Job drawing, mm, ordinate dimensions from the low corner. One solid piece. A direction names the side the tool comes from. Round coordinates to 2 decimals unless told otherwise and drop trailing zeros. Write each loop counter-clockwise with the first axis right and the second up, starting at its lowest first coordinate (ties: lowest second). Pieces come first, ordered by that corner, then holes.
1) Saw through at A-A (x = 15). Write the cut outline in (y, z).
2) Wall check: probe 1 along Z at (x, y) = (15, 26.5); probe 2 along X at (y, z) = (7, 7); probe 3 along Y at (x, z) = (1.5, 4.5). Give the ranges that are in metal, low to high.
3) Which spindle directions (+Z, -Z, +X, -X, +Y, -Y) get a long thin tool onto all of the face, cutting with end or side? Do the marked faces 1 and 2. Say none if no direction does.
4) Saw through at B-B (z = 34.5). Write the cut outline in (x, y), plus the area to 3 significant figures.
5) Saw through at C-C (y = 29). Write the cut outline in (x, z).
6) Flat gauge pins, fed straight in: pin 1 (5.5 mm diameter, centred on x = 11, z = 18, fed in from -Y); pin 2 (12 mm diameter, centred on y = 14.5, z = 12.5, fed in from -X). Where does each tip first touch, or does it go through?
7) Saw through at D-D (z = 29). Write the cut outline in (x, y).
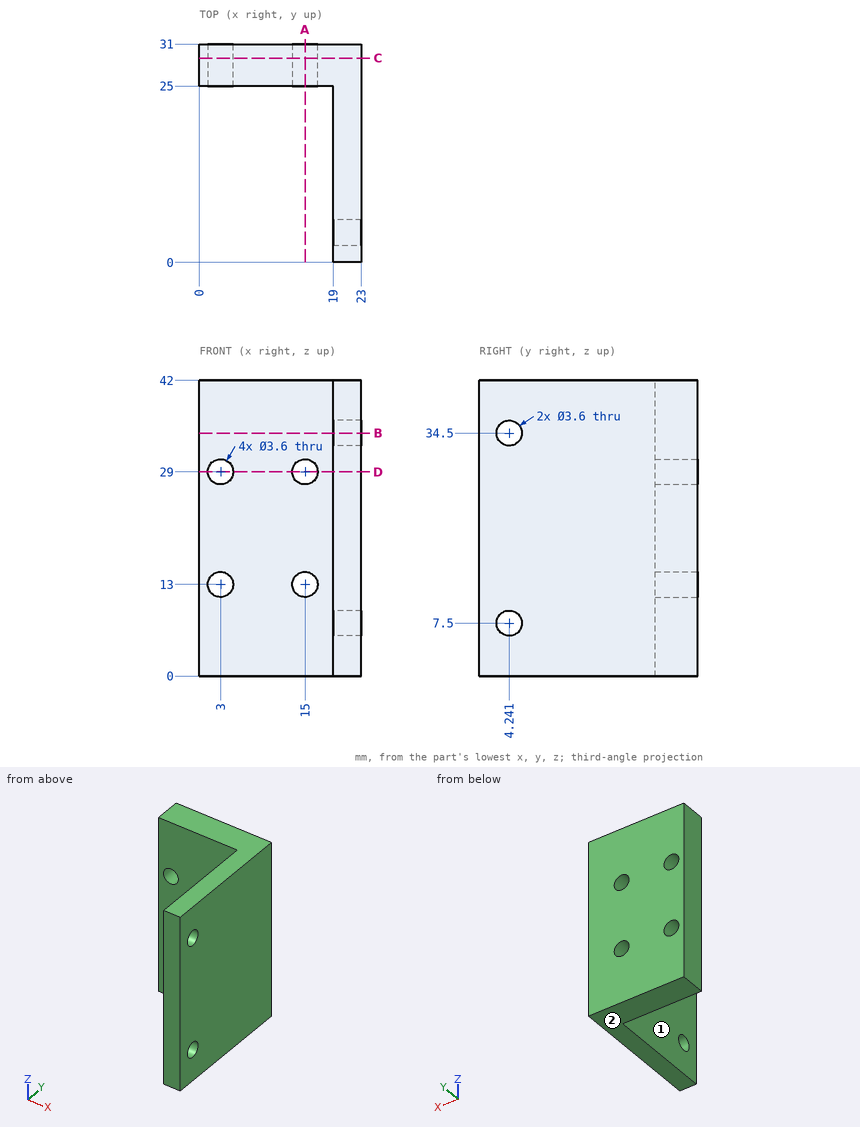
Evaluation:
1. outline: (25, 0) - (31, 0) - (31, 11.2) - (25, 11.2) - close; (25, 14.8) - (31, 14.8) - (31, 27.2) - (25, 27.2) - close; (25, 30.8) - (31, 30.8) - (31, 42) - (25, 42) - close
2. probe 1: z = 0 to 11.2, 14.8 to 27.2, 30.8 to 42
2. probe 2: x = 19 to 23
2. probe 3: y = 25 to 31
3. face 1: +Z, -Z, -X, -Y
3. face 2: -Z, +X, -X, +Y, -Y
4. outline: (0, 25) - (19, 25) - (19, 6.04) - (23, 6.04) - (23, 31) - (0, 31) - close; (19, 0) - (23, 0) - (23, 2.44) - (19, 2.44) - close
4. area: 224 mm2
5. outline: (0, 0) - (23, 0) - (23, 42) - (0, 42) - close; hole circle Ø3.6 at (3, 13); hole circle Ø3.6 at (3, 29); hole circle Ø3.6 at (15, 13); hole circle Ø3.6 at (15, 29)
6. pin 1: stops at y = 25
6. pin 2: stops at x = 19
7. outline: (0, 25) - (1.2, 25) - (1.2, 31) - (0, 31) - close; (4.8, 25) - (13.2, 25) - (13.2, 31) - (4.8, 31) - close; (16.8, 25) - (19, 25) - (19, 0) - (23, 0) - (23, 31) - (16.8, 31) - close
